The drawing under review shows one solid part. Ordinate dimensions are in mm from its lowest x, y, z. Coordinates: 2 decimals unless noted, no trailing zeros. Write each loop counter-clockwise with the first axis right and the second up, starting at its lowest first coordinate (ties: lowest second). Pieces come first, ordered by that corner, then holes. Notation, with made-up numbers: (75, 11.25) - (102, 11.25) arc R18 cw to (102, 19.25) - close; hole circle Ø2 at (21, -12). An arc over 180 degrees is marked (long way). Put each result on its own line as item: value. Start each with the question number.
Item 1: Consider section C-C on x = 4. Give the boundary of the cut face in (y, z).
Item 2: For pin 1 (1.5 mm diameter, centred on y = 12, z = 3, fed in from -X), flat-tipped, find the tip position at first contact; note if it passes through.
Item 3: Mouldability with a two-part tool opening along X and no side actions: class the marked faces 1, 2, 3 and 4 as pulls with the +X half, pulls with the -X half, needs draft (parallel to the pull), parting line crosses it, or undercut.
Item 4: Consider section A-A on x = 10. Give the boundary of the cut face in (y, z).
Item 5: Consider section B-B on z = 7. Give the boundary of the cut face in (x, y).
Item 6: To check wall thickness, follow L1, parallel to Y at x = 10, z = 6.35; L2, parallel to X at y = 9, z = 3.5; L3, parallel to X at y = 8.5, z = 3.5. State the ranges of each line that lie inside material, in increasing order. Write a range as [from, to].
Item 7: Consider section D-D on y = 3.25. Give the boundary of the cut face in (x, z), then the cut area to 3 significant figures.
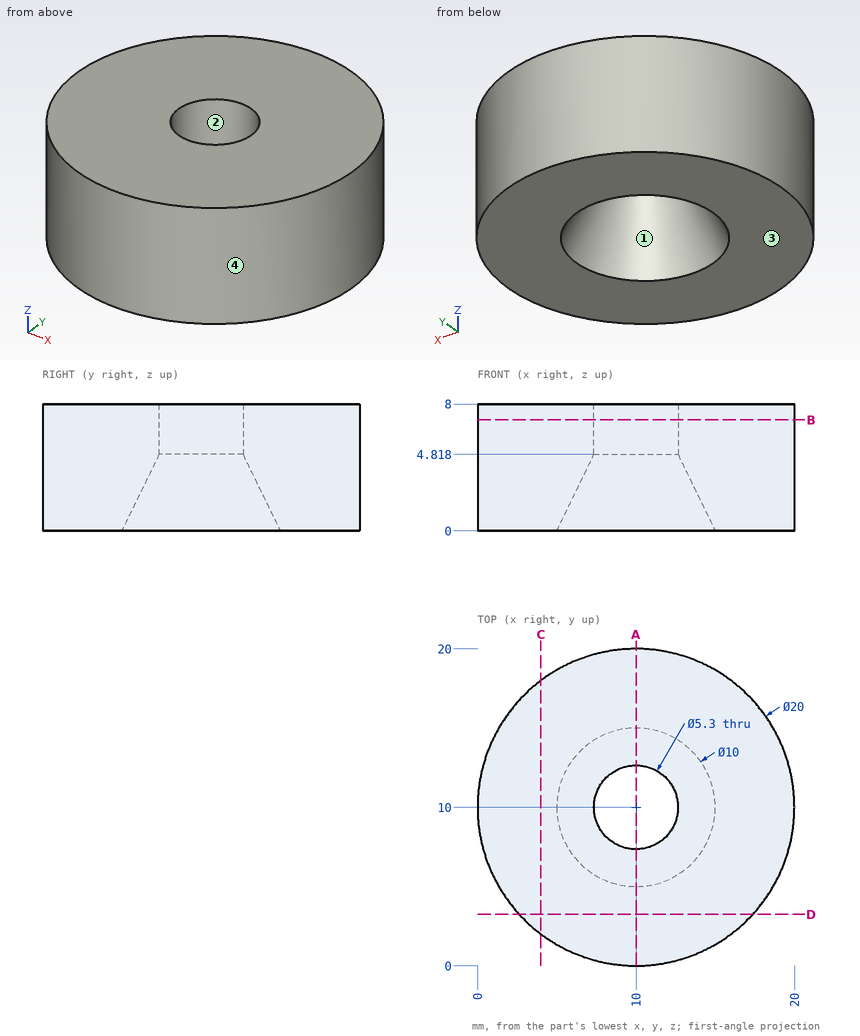
Report:
1. outline: (2, 0) - (18, 0) - (18, 8) - (2, 8) - close
2. pin 1: x = 0.08
3. face 1: undercut
3. face 2: undercut
3. face 3: needs draft
3. face 4: parting line crosses it
4. outline: (0, 0) - (5, 0) - (7.35, 4.82) - (7.35, 8) - (0, 8) - close; (12.65, 4.82) - (15, 0) - (20, 0) - (20, 8) - (12.65, 8) - close
5. outline: circle Ø20 at (10, 10); hole circle Ø5.3 at (10, 10)
6. L1: [0, 7.35], [12.65, 20]
6. L2: [0.05, 6.86], [13.14, 19.95]
6. L3: [0.11, 7.07], [12.93, 19.89]
7. outline: (2.62, 0) - (17.38, 0) - (17.38, 8) - (2.62, 8) - close
7. area: 118 mm²
